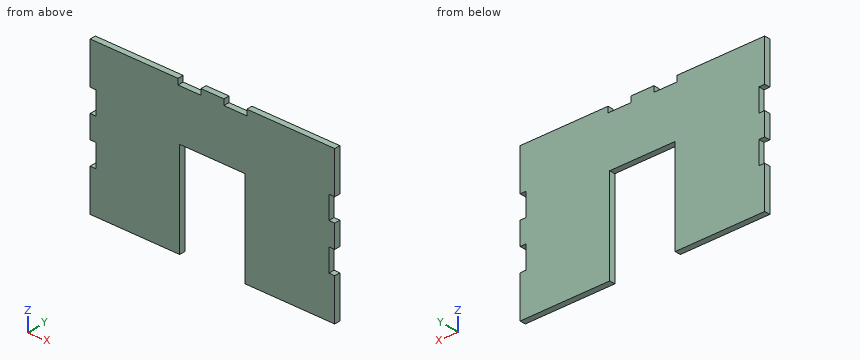
```python
from build123d import *

# Parameters (mm, degrees)
SKETCH1_W        = 203.2
SKETCH1_H        = 177.8
BASE_DEPTH       = 4.826
SKETCH5_W        = 203.2
SKETCH5_H        = 50.8
TRIM_DEPTH       = 271.048829429
SKETCH3_W        = 54.356
SKETCH3_H        = 79.756
CENTER_CUT_DEPTH = 240.67171355
SKETCH2_W        = 4.826
SKETCH2_H        = 19.05
SIDE_SLOTS_DEPTH = 240.67171355
SKETCH4_W        = 19.05
SKETCH4_H        = 4.826
REAR_SLOTS_DEPTH = 240.67171355


with BuildPart() as part:
    # Sketch1 → Base (new body)
    with BuildSketch(Plane(origin=(0, 0, 0), x_dir=(1, 0, 0), z_dir=(0, 1, 0))):
        with Locations((101.6, 88.9)):
            Rectangle(SKETCH1_W, SKETCH1_H)
    extrude(amount=BASE_DEPTH)

    # Sketch5 → Trim (cut, through all)
    with BuildSketch(Plane(origin=(0, 4.826, 0), x_dir=(1, 0, 0), z_dir=(0, 1, 0))):
        with Locations((101.6, 152.4)):
            Rectangle(SKETCH5_W, SKETCH5_H)
    extrude(amount=-TRIM_DEPTH, mode=Mode.SUBTRACT)

    # Sketch3 → Center Cut (cut, through all)
    with BuildSketch(Plane(origin=(0, 4.826, 0), x_dir=(1, 0, 0), z_dir=(0, 1, 0))):
        with Locations((101.6, 87.122)):
            Rectangle(SKETCH3_W, SKETCH3_H)
    extrude(amount=-CENTER_CUT_DEPTH, mode=Mode.SUBTRACT)

    # Sketch2 → Side Slots (cut, through all)
    with BuildSketch(Plane(origin=(0, 4.826, 0), x_dir=(1, 0, 0), z_dir=(0, 1, 0))):
        with Locations((2.413, 82.55)):
            Rectangle(SKETCH2_W, SKETCH2_H)
        with Locations((2.413, 44.45)):
            Rectangle(SKETCH2_W, SKETCH2_H)
        with Locations((200.787, 44.45)):
            Rectangle(SKETCH2_W, SKETCH2_H)
        with Locations((200.787, 82.55)):
            Rectangle(SKETCH2_W, SKETCH2_H)
    extrude(amount=-SIDE_SLOTS_DEPTH, mode=Mode.SUBTRACT)

    # Sketch4 → Rear Slots (cut, through all)
    with BuildSketch(Plane(origin=(0, 4.826, 0), x_dir=(1, 0, 0), z_dir=(0, 1, 0))):
        with Locations((82.55, 2.413)):
            Rectangle(SKETCH4_W, SKETCH4_H)
        with Locations((120.65, 2.413)):
            Rectangle(SKETCH4_W, SKETCH4_H)
    extrude(amount=-REAR_SLOTS_DEPTH, mode=Mode.SUBTRACT)


solid = part.part
```
Check sheet for the modelled part. Datum: model origin and axes. Units: mm. Give positions to 0.01 mm unless a question says otherwise; leave off trailing zeros. Order: outer loops, then holes, each group sorted by start corner. A loop starts at its lowest first (then second) coordinate and runs counter-clockwise, first axis right, second up. Notation, with made-up numbers: (19, 27.25) -> (60, 27.25) arc R22 ccw to (60, 42.25) -> close; hole circle Ø9 at (46, 18.5). An arc over 180 degrees is marked (long way). Return JSON: item names as keys, results as strings.
1. Material ranges on probe 1 along X at (y, z) = (3.5, -65); probe 2 along X at (y, z) = (0.85, -76); probe 3 along Z at (x, y) = (115.5, 1.15), recorded low to high. Write a range as [from, to].
From the geometry:
{"probe 1": "[0, 74.42], [128.78, 203.2]", "probe 2": "[4.83, 74.42], [128.78, 198.37]", "probe 3": "[-47.24, -4.83]"}
2. Cross-section at C-C, the plane x = 123. Record the cut outline in (y, z), plus the area to 3 significant figures.
From the geometry:
{"outline": "(0, -47.24) -> (4.83, -47.24) -> (4.83, -4.83) -> (0, -4.83) -> close", "area": "205 mm^2"}
3. Cross-section at A-A, the plane z = -78.5. Record the cut outline in (x, y).
From the geometry:
{"outline": "(4.83, 0) -> (74.42, 0) -> (74.42, 4.83) -> (4.83, 4.83) -> close; (128.78, 0) -> (198.37, 0) -> (198.37, 4.83) -> (128.78, 4.83) -> close"}
4. Go/stop test with flat-tipped pins: P1, Ø2, axis at y = 4, z = -83, coming from the +X side; P2, Ø1.4, axis at x = 84.5, y = 2, coming from the +Z side; P3, Ø2.5, axis at y = 1.5, z = -79.5, coming from the -X side. Record where each tip stops, or that it passes through.
From the geometry:
{"P1": "x = 198.37", "P2": "z = -4.83", "P3": "x = 4.83"}
5. Cross-section at D-D, the plane z = -115.5. Record the cut outline in (x, y), plus the area to 3 significant figures.
From the geometry:
{"outline": "(0, 0) -> (74.42, 0) -> (74.42, 4.83) -> (0, 4.83) -> close; (128.78, 0) -> (203.2, 0) -> (203.2, 4.83) -> (128.78, 4.83) -> close", "area": "718 mm^2"}
